Read the model definition and answer for the solid it produces. Units are mm, in the model's axes. A direction names the side the tool comes from. Coordinates: 2 decimals unless noted, no trailing zeros. Write each loop counter-clockwise with the first axis right and the second up, starting at its lowest first coordinate (ties: lowest second). Pieces come first, ordered by that corner, then holes.
(1) Section C-C on x = 7 is taken. Write down the section's boundary in (y, z).
(2) The mould has two halves that part along X. Classify faces 6 (the flat face through (-7.46, 69.79, 12.52)), 7 (the cylindrical face through (4.509, 44.783, 12.522)), 8 (the flat face through (3.381, 58, 13)), 9 (the cylindrical face through (-0.3, -8.49, 12.52)): +X half, -X half, draft (parallel to the pull), parting line (faces both ways), or undercut.
(3) Section B-B on z = 16.75 is taken. Write down the section's boundary in (x, y).
(4) Given pin 1 (1.3 mm diameter, centred on y = 33.5, z = 17, fed in from -X); pin 2 (10 mm diameter, centred on y = 43, z = 5.5, fed in from -X); pin 3 (1 mm diameter, centred on y = 65, z = 5.5, fed in from -X), each flat-ended and moving along its own axis, determine where each tip first touches the part or whether it passes through.
(5) Section D-D on y = 58 is taken. Write down the section's boundary in (x, z).
(6) Which of the six approach directions +Z, -Z, +X, -X, +Y, -Y give full straight-line access (tool end or side, diameter ignored) to faces 1 (the flat face through (5.196, 74.283, 12.522)), 2 (the flat face through (-3, 25, 25.4)), 3 (the flat face through (4.083, 19, 13)), 4 (the flat face through (8.37, 69.09, 12.52)), 5 (the flat face through (-2.833, 58, 13))?
(7) Find the intervals of material crossed by probe 1 along X at (y, z) = (30.5, 16); probe 2 along X at (y, z) = (31.5, 8.25); probe 3 along Y at (x, z) = (7.25, 8), in increasing order.
(8) Section A-A on y = 19 is taken. Write down the section's boundary in (x, z), then the cut area to 3 significant figures.
from build123d import *

# Parameters (mm, degrees)
F0_R     = 3.472863
F0_R_2   = 3.604179
F1_DEPTH = 25.4


with BuildPart() as f1:
    # F0 (on Top) → F1 (new body)
    with BuildSketch(Plane.XY):
        with BuildLine():
            Line((13.202485, 5.667426), (13.202485, 35.130091))
            ThreePointArc((13.202485, 35.130091), (10.662539, 43.570376), (3.380966, 48.537108))
            Line((3.380966, 48.537108), (3.380966, 67.268364))
            Line((3.380966, 67.268364), (13.493051, 70.964341))
            Line((13.493051, 70.964341), (10.24771, 76.999515))
            Line((10.24771, 76.999515), (0, 71.488935))
            Line((0, 71.488935), (-9.516433, 76.70256))
            Line((-9.516433, 76.70256), (-11.954483, 72.252385))
            Line((-11.954483, 72.252385), (-2.833481, 67.2554))
            Line((-2.833481, 67.2554), (-2.833481, 48.669556))
            ThreePointArc((-2.833481, 48.669556), (-10.490695, 43.799697), (-13.202949, 35.139897))
            Line((-13.202949, 35.139897), (-13.202949, 5.660794))
            ThreePointArc((-13.202949, 5.660794), (0.003324, -8.493987), (13.202485, 5.667426))
        make_face()
        Polygon((-2.082214, 31.106506), (-9.516433, 31.106506), (-9.516433, 35.272334), (10.24771, 35.095599), (10.24771, 30.74386), (4.08275, 30.74386), (4.08275, 6.446655), (-2.082214, 6.446655), align=None, mode=Mode.SUBTRACT)
        with Locations((-4.979815, 41.006282)):
            Circle(F0_R, mode=Mode.SUBTRACT)
        with Locations((4.978646, 41.209515)):
            Circle(F0_R_2, mode=Mode.SUBTRACT)
    extrude(amount=F1_DEPTH)


solid = f1.part
Response:
1. outline: (-6.49, 0) - (30.74, 0) - (30.74, 25.4) - (-6.49, 25.4) - close; (35.12, 0) - (38.23, 0) - (38.23, 25.4) - (35.12, 25.4) - close; (44.19, 0) - (46.97, 0) - (46.97, 25.4) - (44.19, 25.4) - close; (68.59, 0) - (75.25, 0) - (75.25, 25.4) - (68.59, 25.4) - close
2. face 6: -X half
2. face 7: undercut
2. face 8: +X half
2. face 9: parting line
3. outline: (-13.2, 5.66) arc R13.23 ccw (long way) to (13.2, 5.67) - (13.2, 35.13) arc R13.22 ccw to (3.38, 48.54) - (3.38, 67.27) - (13.49, 70.96) - (10.25, 77) - (0, 71.49) - (-9.52, 76.7) - (-11.95, 72.25) - (-2.83, 67.26) - (-2.83, 48.67) arc R13.22 ccw to (-13.2, 35.14) - close; hole (-9.52, 31.11) - (-2.08, 31.11) - (-2.08, 6.45) - (4.08, 6.45) - (4.08, 30.74) - (10.25, 30.74) - (10.25, 35.1) - (-9.52, 35.27) - close; hole circle Ø6.95 at (-4.98, 41.01); hole circle Ø7.21 at (4.98, 41.21)
4. pin 1: stops at x = -13.2
4. pin 2: stops at x = -13.03
4. pin 3: stops at x = -2.83
5. outline: (-2.83, 0) - (3.38, 0) - (3.38, 25.4) - (-2.83, 25.4) - close
6. face 1: +Z, -Z, +Y
6. face 2: +Z, +X, -X, +Y, -Y
6. face 3: +Z, -Z
6. face 4: +Z, -Z, +X
6. face 5: +Z, -Z, -X
7. probe 1: x = -13.2 to -2.08, 4.08 to 13.2
7. probe 2: x = -13.2 to -9.52, 10.25 to 13.2
7. probe 3: y = -6.33 to 30.74, 35.12 to 38.41, 44.01 to 46.81, 68.68 to 75.39
8. outline: (-13.2, 0) - (-2.08, 0) - (-2.08, 25.4) - (-13.2, 25.4) - close; (4.08, 0) - (13.2, 0) - (13.2, 25.4) - (4.08, 25.4) - close
8. area: 514 mm2
